For this review, take the finished solid that the model builds, in its own axes (mm). A direction names the side the tool comes from. Give positions to 0.01 mm unless a question says otherwise; leave off trailing zeros. Order: outer loops, then holes, each group sorted by start corner. A loop starts at its lowest first (then second) coordinate and runs counter-clockwise, first axis right, second up. Notation, with made-up numbers: M 29,61 L 52,61 A20 ccw 52,87 Z; hole C -7,15.25 d10. An arc over 180 degrees is marked long. Use CSV: the item, a comma, the result in double quotes. Start each with the question number.
(1) Clearance check with flat-ended pins moving along their axes: P1, Ø2.5, axis at x = 31.5, y = 45, coming from the -Z side; P2, Ø10, axis at x = 43.5, z = -8, coming from the -Y side; P3, Ø3, axis at x = 36.5, z = -10, coming from the +Y side; P4, Ø1.5, axis at x = 22.5, z = -9, coming from the -Y side. State where each tip first meets the part, or that it passes through.
(2) Consider section A-A (y = -2.5). Write out the cut boundary in (x, z).
(3) Consider section D-D (x = 31.5). Write out the cut boundary in (y, z).
(4) Wall thickness on L1, parallel to Y at x = 25, z = -2.25; L2, parallel to Z at x = 28.5, y = -24; L3, parallel to Y at x = 38.5, z = 11: over which ranges is each line inside the solid? List them lowest first. Write a range as from..to.
(5) Draft analysis for pull direction Z (two halves, no side actions). For faces 4 (the face through (15, 42, 17)), 5 (the face through (25, -35, -12)), 6 (the face through (25, 42, 13)), 7 (the face through (0, 4, 1)), state which applies: pulls with the +Z half, pulls with the -Z half, needs draft (parallel to the pull), parting line crosses it, or undercut.
(6) Consider section B-B (x = 25). Write out the cut boundary in (y, z).
(7) Tool access review of faces 1 (the face through (25, 9, 6)), 2 (the face through (25, -22.5, -12)), 3 (the face through (30, 42, 25)): name each direction out of +Z, -Z, +X, -X, +Y, -Y from which nothing blocks a thin tool from reaching the whole face with its end or side.
(8) Consider section C-C (z = -4). Write out the cut boundary in (x, y), and give its area (3 significant figures).
```python
from build123d import *

# Parameters (mm, degrees)
F1_DEPTH = 50
F3_DEPTH = 25
F4_R     = 9
F5_DEPTH = 25


with BuildPart() as f1:
    # F0 (on Right) → F1 (new body)
    with BuildSketch(Plane.YZ):
        Polygon((37.5, -6), (37.5, 6), (-37.5, 6), (-37.5, -6), (-22.5, -6), align=None)
        Polygon((37.5, 29), (37.5, 6), (37.5, -6), (47.5, -6), (47.5, 29), align=None)
        Polygon((-22.5, -6), (-37.5, -6), (-32.5, -18), (-22.5, -18), align=None)
    extrude(amount=F1_DEPTH)

    # F2 (on face) → F3 (cut)
    with BuildSketch(Plane.XZ.offset(-37.5)):
        Polygon((30, 29), (20, 29), (20, 21), (15, 21), (15, 13), (35, 13), (35, 21), (30, 21), align=None)
    extrude(amount=-F3_DEPTH, mode=Mode.SUBTRACT)

    # F4 (on face) → F5 (cut)
    with BuildSketch(Plane.XY.offset(6)):
        with Locations((25, -2.5)):
            Circle(F4_R)
    extrude(amount=-F5_DEPTH, mode=Mode.SUBTRACT)


solid = f1.part
```
Check result:
1,P1,"stops at z = -6"
1,P2,"stops at y = -37.5"
1,P3,"stops at y = -22.5"
1,P4,"stops at y = -36.56"
2,outline,"M 0,-6 L 16,-6 L 16,6 L 0,6 Z; M 34,-6 L 50,-6 L 50,6 L 34,6 Z"
3,outline,"M -37.5,-6 L -32.5,-18 L -22.5,-18 L -22.5,-6 L -8.72,-6 L -8.72,6 L -37.5,6 Z; M 3.72,-6 L 47.5,-6 L 47.5,13 L 37.5,13 L 37.5,6 L 3.72,6 Z; M 37.5,21 L 47.5,21 L 47.5,29 L 37.5,29 Z"
4,L1,"y = -37.5..-11.5, 6.5..47.5"
4,L2,"z = -18..6"
4,L3,"y = 37.5..47.5"
5,face 4,"undercut"
5,face 5,"pulls with the -Z half"
5,face 6,"undercut"
5,face 7,"needs draft"
6,outline,"M -37.5,-6 L -32.5,-18 L -22.5,-18 L -22.5,-6 L -11.5,-6 L -11.5,6 L -37.5,6 Z; M 6.5,-6 L 47.5,-6 L 47.5,13 L 37.5,13 L 37.5,6 L 6.5,6 Z"
7,face 1,"+Z, +X, -X, -Y"
7,face 2,"-Z, +X, -X, +Y"
7,face 3,"+Z, +Y, -Y"
8,outline,"M 0,-37.5 L 50,-37.5 L 50,47.5 L 0,47.5 Z; hole C 25,-2.5 d18"
8,area,"4,000 mm^2"
